Here's how the part is built. I have some questions about the finished solid (model axes, mm). A direction names the side the tool comes from. Round coordinates to 2 decimals unless told otherwise and drop trailing zeros. Write each loop counter-clockwise with the first axis right and the second up, starting at its lowest first coordinate (ties: lowest second). Pieces come first, ordered by that corner, then holes. Notation, with made-up numbers: (78.5, 57) - (128.5, 57) arc R23 ccw to (128.5, 87) - close; hole circle Ø4 at (-35, 12). An arc over 180 degrees is marked (long way). One line per item, written item: value. Start each with the question number.
Item 1: Imagine slicing it at A-A, the plane z = -10. Please give me the cut outline in (x, y), then the cut area to 3 significant figures.
Item 2: Thinking about a two-plate mould opening in Y: for faces 1 (the face through (5.92, 18.43, -19.72)), 2 (the face through (5.92, -3.67, 35.27)), 3 (the face through (6.084, 23.626, -25.446)), which applies, released by +Y, released by -Y, zero draft, split by the parting line, or undercut?
Item 3: Imagine slicing it at C-C, the plane z = 26.5. Please give me the cut outline in (x, y), then the cut area to 3 significant figures.
Item 4: Imagine slicing it at D-D, the plane y = 30. Please give me the cut outline in (x, z).
Item 5: Imagine slicing it at B-B, the plane x = 10.5. Count the separate pieces of the cut face and the enclosed holes in it, then the cut area to 3 significant figures.
Item 6: For P1, Ø2, axis at x = 8.5, y = 6, coming from the -Z side; P2, Ø8, axis at y = 33.5, z = -28, coming from the +X side; P3, Ø4, axis at x = 9.5, y = 23.5, coming from the -Z side; P4, Ø1.5, axis at x = 1.5, y = 13.5, coming from the -Z side, each with a flat end and sliding along its axis, tell me the tip position at first contact or that it passes through.
Item 7: If I drill on line 1 (X direction, y = 43.45, z = 10); line 2 (Z direction, x = 7.5, y = 15); line 3 (Z direction, x = 7, y = 30), over which ranges is the centre line in solid material (lowest first)?
Item 8: For faces 4 (the face through (6.084, 22.377, 21.578)), 5 (the face through (12, 40.3, -0.2)), 6 (the face through (6.084, 39.517, -15.619)), which set-ups out of +Z, -Z, +X, -X, +Y, -Y let a thin tool reach every point of the face, with its end or its side?
```python
from build123d import *

# Parameters (mm, degrees)
SKETCH1_R           = 7
SKETCH1_R_2         = 5
BOSS_EXTRUDE1_DEPTH = 12
CUT_EXTRUDE1_DEPTH  = 40.522145691
FILLET1_R           = 1
BOSS_EXTRUDE2_START = -12
BOSS_EXTRUDE2_DEPTH = 12
FILLET2_R           = 2
CUT_EXTRUDE2_DEPTH  = 59.481408086
SKETCH7_R           = 1.5
CUT_EXTRUDE3_DEPTH  = 65.024019647


with BuildPart() as part:
    # Sketch1 → Boss-Extrude1 (new body)
    with BuildSketch(Plane(origin=(0, 0, 0), x_dir=(0, 0, -1), z_dir=(1, 0, 0))):
        with Locations((-30, 0)):
            Circle(SKETCH1_R)
        with Locations((-30, 0)):
            Circle(SKETCH1_R_2, mode=Mode.SUBTRACT)
    extrude(amount=BOSS_EXTRUDE1_DEPTH)

    # Sketch3 → Cut-Extrude1 (cut, through all)
    with BuildSketch(Plane(origin=(12, 0, 0), x_dir=(0, 0, -1), z_dir=(1, 0, 0))):
        Polygon((-26.132418273, 3.168881756), (-27.092472621, -4.067712446), (-40.54775296, -2.282646151), (-39.587698612, 4.953948051), align=None)
    extrude(amount=-CUT_EXTRUDE1_DEPTH, mode=Mode.SUBTRACT)

    # Fillet1
    fillet1_edges = [part.edges().sort_by_distance(p)[0] for p in [
        (6, 4.067712446, 32.907527379),
        (6, 4.403840469, 35.441156966),
        (6, -3.168881756, 33.867581727),
        (6, -2.832753733, 36.401211314),
    ]]
    fillet(fillet1_edges, radius=FILLET1_R - 0.0001)  # a hair under: the kernel refuses the full size

    # Sketch4 → Boss-Extrude2 (add)
    with BuildSketch(Plane(origin=(12, 0, 0), x_dir=(0, 0, -1), z_dir=(1, 0, 0)).offset(BOSS_EXTRUDE2_START)):
        with BuildLine():
            Line((-23.06080008, -0.92060006), (-16, 40))
            Line((-16, 40), (0, 40))
            Line((0, 40), (0, 45))
            Line((0, 45), (-22, 45))
            Line((-22, 45), (-32.927058907, 6.358641848))
            ThreePointArc((-32.927058907, 6.358641848), (-25.844141537, 5.632835914), (-23.06080008, -0.92060006))
        make_face()
    extrude(amount=BOSS_EXTRUDE2_DEPTH)

    # Fillet2
    fillet2_edges = [part.edges().sort_by_distance(p)[0] for p in [
        (6, 40, 16),
    ]]
    fillet(fillet2_edges, radius=FILLET2_R)

    # Sketch6 → Cut-Extrude2 (cut, through all)
    with BuildSketch(Plane(origin=(12, 0, 0), x_dir=(0, 0, -1), z_dir=(1, 0, 0))):
        with BuildLine():
            Line((-23.744298761, 9.820968741), (-19.349752742, 35.289394134))
            ThreePointArc((-19.349752742, 35.289394134), (-20.381234985, 36.835447129), (-21.979152767, 35.886292641))
            Line((-21.979152767, 35.886292641), (-29.011800399, 11.016740989))
            ThreePointArc((-29.011800399, 11.016740989), (-27.008090108, 7.643460534), (-23.744298761, 9.820968741))
        make_face()
    extrude(amount=-CUT_EXTRUDE2_DEPTH, mode=Mode.SUBTRACT)

    # Mirror9: part across plane


with BuildPart() as part_1:
    add(part.part)
    add(part.part.mirror(Plane(origin=(-56.505687485, 40, 0), x_dir=(1, 0, 0), z_dir=(0, 0, -1))))

    # Sketch7 → Cut-Extrude3 (cut, through all)
    with BuildSketch(Plane(origin=(0, 45, 0), x_dir=(1, 0, 0), z_dir=(0, 1, 0))):
        with Locations(Location((6, -10, 0), (0, 0, 270))):
            Circle(SKETCH7_R)
        with Locations(Location((6, 10, 0), (0, 0, 270))):
            Circle(SKETCH7_R)
    extrude(amount=-CUT_EXTRUDE3_DEPTH, mode=Mode.SUBTRACT)


solid = part_1.part
```
Values follow:
1. outline: (0, 40) - (4.5, 40) - (4.5, 45) - (0, 45) - close; (7.5, 40) - (12, 40) - (12, 45) - (7.5, 45) - close
1. area: 45.0 mm^2
2. face 1: released by -Y
2. face 2: split by the parting line
2. face 3: undercut
3. outline: (0, -6.06) - (12, -6.06) - (12, -3.57) - (0, -3.57) - close; (0, 3.57) - (12, 3.57) - (12, 7.58) - (0, 7.58) - close; (0, 19.9) - (12, 19.9) - (12, 29.09) - (0, 29.09) - close
3. area: 188 mm^2
4. outline: (0, -26.24) - (12, -26.24) - (12, -23.64) - (0, -23.64) - close; (0, -20.26) - (12, -20.26) - (12, -17.73) - (0, -17.73) - close; (0, 17.73) - (12, 17.73) - (12, 20.26) - (0, 20.26) - close; (0, 23.64) - (12, 23.64) - (12, 26.24) - (0, 26.24) - close
5. separate pieces: 1
5. enclosed holes: 2
5. area: 745 mm^2
6. P1: stops at z = -34.15
6. P2: stops at x = 12
6. P3: stops at z = -28.65
6. P4: stops at z = -31.12
7. line 1: x = 0 to 4.5, 7.5 to 12
7. line 2: z = -30.48 to -27.89, -22.85 to -20.31, 20.31 to 22.85, 27.89 to 30.48
7. line 3: z = -26.24 to -23.64, -20.26 to -17.73, 17.73 to 20.26, 23.64 to 26.24
8. face 4: +X, -X
8. face 5: +Z, -Z, +X, +Y, -Y
8. face 6: +X, -X, -Y
